```python
from build123d import *

# Parameters (mm, degrees)
F0_R     = 8.0316205534
F2_R     = 14.2875
F4_R     = 14.2875
F8_D     = 12.04743083
F8_DEPTH = 38.1
F8_TIP   = 3.6194133731
F9_SIZE2 = 2.9329393675
F9_SIZE  = 5.08


with BuildPart() as f5:
    # F0 (on Top) → F5 section 0
    with BuildSketch(Plane.XY):
        Circle(F0_R)
    # F2 (on offset) → F5 section 1
    with BuildSketch(Plane.XY.offset(12.7)):
        Circle(F2_R)
    loft()

    # F4 (on offset) → F6 section 0
    with BuildSketch(Plane.XY.offset(63.5)):
        Circle(F4_R)
    # F2 (on offset) → F6 section 1
    with BuildSketch(Plane.XY.offset(12.7)):
        Circle(F2_R)
    loft()

    # F8
    with Locations(Plane(origin=(0, 0, 0), x_dir=(1, 0, 0), z_dir=(0, 0, -1))):
        with Locations((0, 0)):
            Hole(F8_D / 2, depth=F8_DEPTH)
            with Locations((0, 0, -(F8_DEPTH + F8_TIP / 2))):  # 118° drill point
                Cone(0, F8_D / 2, F8_TIP, mode=Mode.SUBTRACT)

    # F9
    f9_edges = [f5.edges().sort_by_distance(p)[0] for p in [
        (-14.2875, 0, 63.5),
    ]]
    chamfer(f9_edges, length=F9_SIZE, length2=F9_SIZE2)


solid = f5.part
```
The listing builds one solid part. Answer for the finished solid, in the listing's coordinates (mm). Give positions to 0.01 mm unless a question says otherwise; leave off trailing zeros. Loops run counter-clockwise (first coordinate to the right, second up) from the corner with the lowest first, then second, coordinate; pieces in that order, holes last. Notation, with made-up numbers: (23.5, 83) - (38.5, 83) arc R24 cw to (38.5, 101) - close; hole circle Ø2 at (-23.75, 1). An arc over 180 degrees is marked (long way). Answer as CSV lines item,"result". Start each with the question number.
Item 1: Find the intervals of material crossed by line 1 (Y direction, x = 0, z = 19); line 2 (X direction, y = -0.25, z = 57.5); line 3 (Y direction, x = 3, z = 34.5), in increasing order. Write a range as from..to.
Item 2: A cutting plane is placed at A-A on z = 30. Determine the outline of the cut face in (x, y) (1 decimal), then the cut area to 3 significant figures.
Item 3: Each of these flat-tipped pins is pushed along its axis until it touches: pin 1 (1.5 mm diameter, centred on y = -0.5, z = 7.5, fed in from -X); pin 2 (1 mm diameter, centred on x = -10.5, z = 12.5, fed in from -Y); pin 3 (8 mm diameter, centred on x = -7, z = 12.5, fed in from +Y). Where does it stop, or does it pass through?
Item 4: A cutting plane is placed at C-C on z = 5. Determine the outline of the cut face in (x, y), then the cut area to 3 significant figures.
Item 5: A cutting plane is placed at B-B on z = 56. Determine the outline of the cut face in (x, y) (1 decimal).
Item 6: The mould has two halves that part along X. Classify faces 1 (the face through (0, 0, 63.5)), 2 (the face through (1.31, 5.88, 19.32)), 3 (the face through (-2.492, -11.224, 63.253)): +X half, -X half, draft (parallel to the pull), parting line (faces both ways), or undercut.
Found:
1,line 1,"y = -14.29..-6.02, 6.02..14.29"
1,line 2,"x = -14.29..14.29"
1,line 3,"y = -13.97..-5.22, 5.22..13.97"
2,outline,"circle Ø28.6 at (0, 0); hole circle Ø12 at (0, 0)"
2,area,"527 mm^2"
3,pin 1,"stops at x = -12.09"
3,pin 2,"stops at y = -10.16"
3,pin 3,"stops at y = 13.97"
4,outline,"circle Ø20.99 at (0, 0); hole circle Ø12.05 at (0, 0)"
4,area,"232 mm^2"
5,outline,"circle Ø28.6 at (0, 0)"
6,face 1,"draft"
6,face 2,"undercut"
6,face 3,"parting line"
